Answer from the drawing. Dimensions are ordinates in mm from the lowest x, y and z of the part. A direction names the side the tool comes from. Round coordinates to 2 decimals unless told otherwise and drop trailing zeros. Loops run counter-clockwise (first coordinate to the right, second up) from the corner with the lowest first, then second, coordinate; pieces in that order, holes last. Notation, with made-up numbers: (81, 11.25) - (97, 11.25) arc R23 cw to (97, 32.25) - close; hole circle Ø7 at (1.5, 45.25). An arc over 180 degrees is marked (long way). Answer as CSV lines item,"result". Start each with the question number.
Q1. The mould has two halves that part along Z. Classify the marked faces 1, 2 and 3: +Z half, -Z half, draft (parallel to the pull), parting line (faces both ways), or undercut.
Q2. Section B-B on y = 38.5 is taken. Write down the section's boundary in (x, z), then the cut area to 3 significant figures.
Q3. Section C-C on z = 57 is taken. Write down the section's boundary in (x, y).
Q4. For the marked faces 4 and 5, determine the directions among +Z, -Z, +X, -X, +Y, -Y from which every point of the face is accessible in a straight line to the end or side of a thin tool.
Q5. Section A-A on x = 50 is taken. Write down the section's boundary in (y, z).
Q6. This flat-tipped pin is pushed along its axis until it touches: pin 1 Ø8 at (x, z) = (28.5, 58) entering from +Y. Where does it stop, or does it pass through?
Q7. Section D-D on x = 10 is taken. Write down the section's boundary in (y, z), then the cut area to 3 significant figures.
Q8. Straight lines are drawn through the part: L1, parallel to X at y = 53, z = 37; L2, parallel to Z at x = 34, y = 60.5; L3, parallel to Y at x = 16, z = 88.5. For each, find the intervals that lie inside material, in ascending order. Write a range as [from, to].
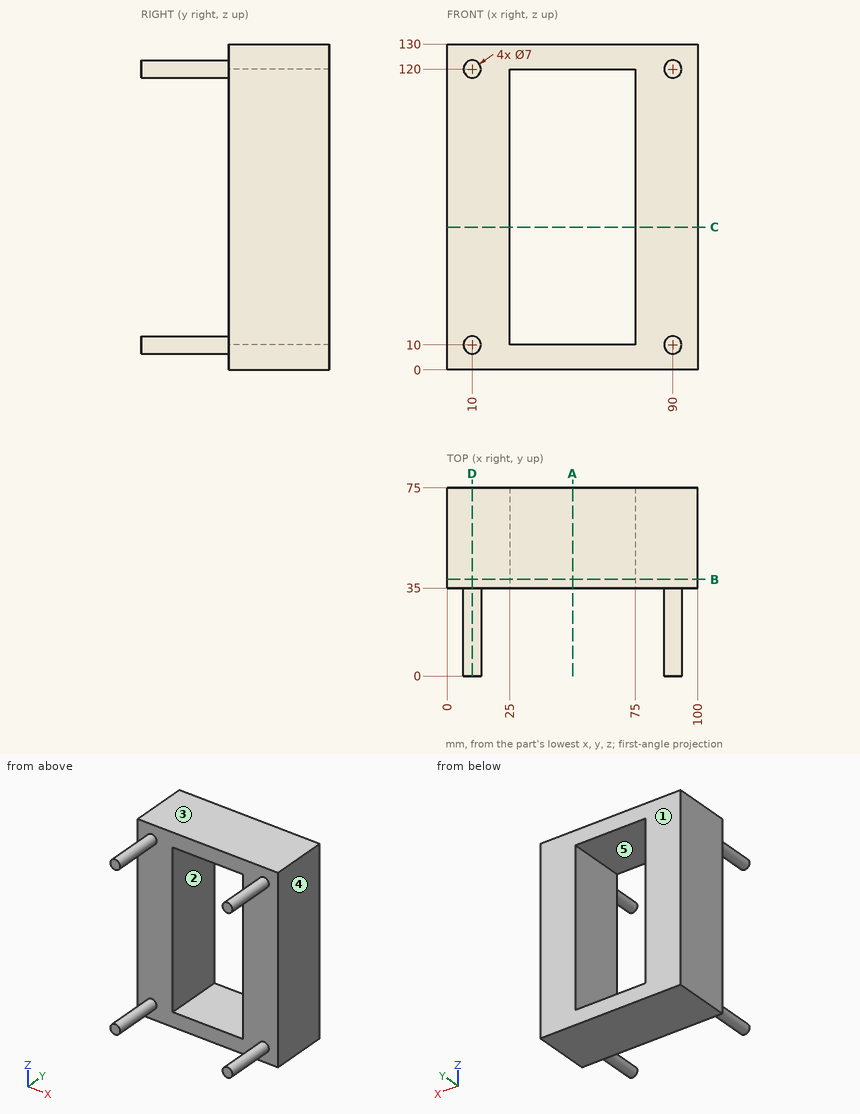
Findings:
1,face 1,"draft"
1,face 2,"undercut"
1,face 3,"+Z half"
2,outline,"(0, 0) - (100, 0) - (100, 130) - (0, 130) - close; hole (25, 10) - (75, 10) - (75, 120) - (25, 120) - close"
2,area,"7,500 mm^2"
3,outline,"(0, 35) - (25, 35) - (25, 75) - (0, 75) - close; (75, 35) - (100, 35) - (100, 75) - (75, 75) - close"
4,face 4,"+Z, -Z, +X, +Y, -Y"
4,face 5,"+Y, -Y"
5,outline,"(35, 0) - (75, 0) - (75, 10) - (35, 10) - close; (35, 120) - (75, 120) - (75, 130) - (35, 130) - close"
6,pin 1,"stops at y = 75"
7,outline,"(0, 6.5) - (35, 6.5) - (35, 0) - (75, 0) - (75, 130) - (35, 130) - (35, 123.5) - (0, 123.5) - (0, 116.5) - (35, 116.5) - (35, 13.5) - (0, 13.5) - close"
7,area,"5,690 mm^2"
8,L1,"x = [0, 25], [75, 100]"
8,L2,"z = [0, 10], [120, 130]"
8,L3,"y = [35, 75]"
